from build123d import *

# Parameters (mm, degrees)
F0_W         = 65
F0_H         = 20
F1_DEPTH     = 7.5
F3_DEPTH     = 2.5
F4_R         = 1.65
F5_DEPTH     = 5
F7_DEPTH     = 3.3
F8_W         = 12
F8_H         = 16
F9_DEPTH     = 2
F10_R        = 1.35
F11_DEPTH    = 5
F12_T4_DEPTH = 16
F15_DEPTH    = 2
F16_DEPTH    = 20
F17_W        = 20
F17_H        = 7.5
F18_DEPTH    = 3
F19_W        = 10.9964999743
F19_H        = 5
F20_DEPTH    = 2
F21_DEPTH    = 1
F22_R        = 5
F23_DEPTH    = 0.5


# Not quite as in the source:
# - a fillet or chamfer that OpenCascade refuses, or shapes differently, is made with other operations: its cross-section is extruded or revolved along the edge and cut away or added


with BuildPart() as f1:
    # F0 (on Top) → F1 (new body)
    with BuildSketch(Plane.XY):
        with Locations((32.5, 10)):
            Rectangle(F0_W, F0_H)
    extrude(amount=F1_DEPTH)

    # F2 (on face) → F3 (cut)
    with BuildSketch(Plane(origin=(0, 0, 0), x_dir=(1, 0, 0), z_dir=(0, 0, -1))):
        Polygon((4.375, -7.8145825623), (7.625, -7.8145825623), (9.25, -5), (7.625, -2.1854174377), (4.375, -2.1854174377), (2.75, -5), align=None)
        Polygon((7.625, -12.1854174377), (4.375, -12.1854174377), (2.75, -15), (4.375, -17.8145825623), (7.625, -17.8145825623), (9.25, -15), align=None)
        Polygon((54.375, -7.8145825623), (57.625, -7.8145825623), (59.25, -5), (57.625, -2.1854174377), (54.375, -2.1854174377), (52.75, -5), align=None)
        Polygon((54.375, -17.8145825623), (57.625, -17.8145825623), (59.25, -15), (57.625, -12.1854174377), (54.375, -12.1854174377), (52.75, -15), align=None)
    extrude(amount=-F3_DEPTH, mode=Mode.SUBTRACT)

    # F4 (on face) → F5 (cut)
    with BuildSketch(Plane(origin=(0, 0, 2.5), x_dir=(1, 0, 0), z_dir=(0, 0, -1))):
        with Locations((6, -5)):
            Circle(F4_R)
        with Locations((6, -15)):
            Circle(F4_R)
        with Locations((56, -5)):
            Circle(F4_R)
        with Locations((56, -15)):
            Circle(F4_R)
    extrude(amount=-F5_DEPTH, mode=Mode.SUBTRACT)

    # F6 (on face) → F7 (cut)
    with BuildSketch(Plane.XY.offset(7.5)):
        Polygon((51, 17.9014432635), (16, 17.9014432635), (16, 12.5), (16, 7.5), (16, 1.9014432635), (51, 1.9014432635), align=None)
        Polygon((16, 12.5), (16, 17.9014432635), (11, 12.5), align=None)
        Polygon((16, 7.5), (16, 12.5), (11, 12.5), (0, 12.5), (0, 7.5), (11, 7.5), align=None)
        Polygon((16, 1.9014432635), (16, 7.5), (11, 7.5), align=None)
    extrude(amount=-F7_DEPTH, mode=Mode.SUBTRACT)

    # F8 (on face) → F9 (cut)
    with BuildSketch(Plane.XY.offset(4.2)):
        with Locations((22, 9.9014432635)):
            Rectangle(F8_W, F8_H)
    extrude(amount=-F9_DEPTH, mode=Mode.SUBTRACT)

    # F10 (on face) → F11 (cut)
    with BuildSketch(Plane.XY.offset(4.2)):
        with Locations((47.8, 14.9014432635)):
            Circle(F10_R)
        with Locations((47.8, 4.9014432635)):
            Circle(F10_R)
    extrude(amount=-F11_DEPTH, mode=Mode.SUBTRACT)

    # F12: chamfer of 5 on 1 edges, made by hand


with BuildPart() as f12_tool2:
    # F12_s3 → F12_t4 (new body)
    with BuildSketch(Plane.XZ.offset(-1.9014432635)):
        Polygon((33, 4.2), (28, -0.8), (28, 4.2), align=None)
    extrude(amount=-F12_T4_DEPTH)

    split(bisect_by=Plane.XY.offset(2.2), keep=Keep.TOP)


with BuildPart() as f1_1:
    add(f1.part)

    # F12_t1: cut F12_tool2
    add(f12_tool2.part, mode=Mode.SUBTRACT)

    # F14 (on face) → F15 (cut)
    with BuildSketch(Plane.XY.offset(4.2)):
        Polygon((16, 17.9014432635), (11, 12.5), (11, 7.5), (16, 1.9014432635), align=None)
    extrude(amount=-F15_DEPTH, mode=Mode.SUBTRACT)

    # F13 (on face) → F16 (join)
    with BuildSketch(Plane.XZ):
        Polygon((10.9964999743, 2.2), (15.9964999743, 2.2), (10.9964999743, 6.2), align=None)
    extrude(amount=-F16_DEPTH)

    # F17 (on face) → F18 (cut)
    with BuildSketch(Plane.YZ.offset(65)):
        with Locations((10, 3.75)):
            Rectangle(F17_W, F17_H)
    extrude(amount=-F18_DEPTH, mode=Mode.SUBTRACT)

    # F19 (on face) → F20 (join)
    with BuildSketch(Plane.XY.offset(4.2)):
        with Locations((5.4982499871, 10)):
            Rectangle(F19_W, F19_H)
    extrude(amount=F20_DEPTH)

    # F21 (add): a face of the model
    f21_faces = [f1_1.faces().sort_by_distance(p)[0] for p in [
        (61.348540101, 10, 7.5),
    ]]
    extrude(f21_faces, amount=F21_DEPTH)

    # F22 (call 1 of 3: OpenCascade refuses the feature's edges together)
    f22_edges = [f1_1.edges().sort_by_distance(p)[0] for p in [
        (11, 12.5, 7.3486),
    ]]
    fillet(f22_edges, radius=F22_R)

    # F22#2 (call 2 of 3)
    f22_2_edges = [f1_1.edges().sort_by_distance(p)[0] for p in [
        (10.9965, 10, 6.2),
    ]]
    fillet(f22_2_edges, radius=F22_R)

    # F22#3 (call 3 of 3)
    f22_3_edges = [f1_1.edges().sort_by_distance(p)[0] for p in [
        (11, 7.5, 7.3486),
    ]]
    fillet(f22_3_edges, radius=F22_R)

    # F23 (cut): a face of the model
    f23_faces = [f1_1.faces().sort_by_distance(p)[0] for p in [
        (51, 9.9014432635, 6.35),
    ]]
    extrude(f23_faces, amount=-F23_DEPTH, mode=Mode.SUBTRACT)


solid = f1_1.part
CAD build for the part. Positions are in the model's coordinates, mm. A direction names the side the tool comes from. Give positions to 0.01 mm unless a question says otherwise; leave off trailing zeros. Order: outer loops, then holes, each group sorted by start corner. A loop starts at its lowest first (then second) coordinate and runs counter-clockwise, first axis right, second up. Notation, with made-up numbers: (50.5, 49) -> (74.5, 49) arc R24 ccw to (74.5, 81) -> close; hole circle Ø7 at (1, 20.25). An arc over 180 degrees is marked (long way). Return JSON: item names as keys, results as strings.
Q1. Which spindle directions (+Z, -Z, +X, -X, +Y, -Y) get a long thin tool onto all of the face, cutting with end or side? Do faces 3 (the face through (46.45, 14.96, 2.13)), 4 (the face through (34, 17.901, 6)), 5 (the face through (53.551, 6.388, 1.232)). Say none if no direction does.
Working result:
{"face 3": "+Z, -Z", "face 4": "+Z", "face 5": "-Z"}
Q2. Saw through at D-D (x = 6). Write the cut outline in (y, z).
Working result:
{"outline": "(0, 0) -> (2.19, 0) -> (2.19, 2.5) -> (3.35, 2.5) -> (3.35, 8.5) -> (0, 8.5) -> close; (6.65, 2.5) -> (7.81, 2.5) -> (7.81, 0) -> (12.19, 0) -> (12.19, 2.5) -> (13.35, 2.5) -> (13.35, 8.5) -> (12.5, 8.5) -> (12.5, 6.2) -> (7.5, 6.2) -> (7.5, 8.5) -> (6.65, 8.5) -> close; (16.65, 2.5) -> (17.81, 2.5) -> (17.81, 0) -> (20, 0) -> (20, 8.5) -> (16.65, 8.5) -> close"}
Q3. Mould opens along X. For faces 1 (the face through (7.4, 16.2, 2.5)), 2 (the face through (58.426, 6.427, 1.232)) say: pulls with the +X half, pulls with the -X half, needs draft (parallel to the pull), parting line crosses it, or undercut.
Working result:
{"face 1": "undercut", "face 2": "undercut"}
Q4. Saw through at A-A (x = 47.8). Write the cut outline in (y, z), then the cut area to 3 significant figures.
Working result:
{"outline": "(0, 0) -> (3.55, 0) -> (3.55, 4.2) -> (1.9, 4.2) -> (1.9, 8.5) -> (0, 8.5) -> close; (6.25, 0) -> (13.55, 0) -> (13.55, 4.2) -> (6.25, 4.2) -> close; (16.25, 0) -> (20, 0) -> (20, 8.5) -> (17.9, 8.5) -> (17.9, 4.2) -> (16.25, 4.2) -> close", "area": "78.5 mm²"}
Q5. Drill centre lines: line 1 (Y direction, x = 47.8, z = 1.8); line 2 (Y direction, x = 6, z = 7); line 3 (Y direction, x = 6, z = 5). Where is each one in solid material? Low to high.
Working result:
{"line 1": "0 to 3.55, 6.25 to 13.55, 16.25 to 20", "line 2": "0 to 3.35, 6.65 to 7.5, 12.5 to 13.35, 16.65 to 20", "line 3": "0 to 3.35, 6.65 to 13.35, 16.65 to 20"}
Q6. Saw through at C-C (x = 26.5). Write the cut outline in (y, z).
Working result:
{"outline": "(0, 0) -> (20, 0) -> (20, 8.5) -> (17.9, 8.5) -> (17.9, 2.2) -> (1.9, 2.2) -> (1.9, 8.5) -> (0, 8.5) -> close"}
Q7. Flat gauge pins, fed straight in: pin 1 (2.5 mm diameter, centred on x = 47.8, y = 4.9, fed in from -Z); pin 2 (1.5 mm diameter, centred on x = 29.5, y = 5, fed in from +Z). Where does each tip first touch, or does it go through?
Working result:
{"pin 1": "through", "pin 2": "z = 2.2"}
Q8. Saw through at B-B (z = 3.25). Write the cut outline in (x, y), then the cut area to 3 significant figures.
Working result:
{"outline": "(0, 0) -> (62, 0) -> (62, 20) -> (0, 20) -> close; hole circle Ø3.3 at (6, 5); hole circle Ø3.3 at (6, 15); hole (14.68, 3.37) -> (16, 1.9) -> (32.05, 1.9) -> (32.05, 17.9) -> (16, 17.9) -> (14.68, 16.48) -> close; hole circle Ø2.7 at (47.8, 4.9); hole circle Ø2.7 at (47.8, 14.9); hole circle Ø3.3 at (56, 5); hole circle Ø3.3 at (56, 15)", "area": "918 mm²"}
